Read the model definition and answer for the solid it produces. Units are mm, in the model's axes. Face numbers are marked on the shaded views. A direction names the side the tool comes from. Coordinates: 2 decimals unless noted, no trailing zeros. Write each loop counter-clockwise with the first axis right and the second up, starting at its lowest first coordinate (ties: lowest second). Pieces come first, ordered by that corner, then holes. Notation, with made-up numbers: (-25, 71.5) - (21, 71.5) arc R32 cw to (21, 97.5) - close; hole circle Ø8 at (-12.75, 53). An arc over 180 degrees is marked (long way). Use a Markdown table: item, result.
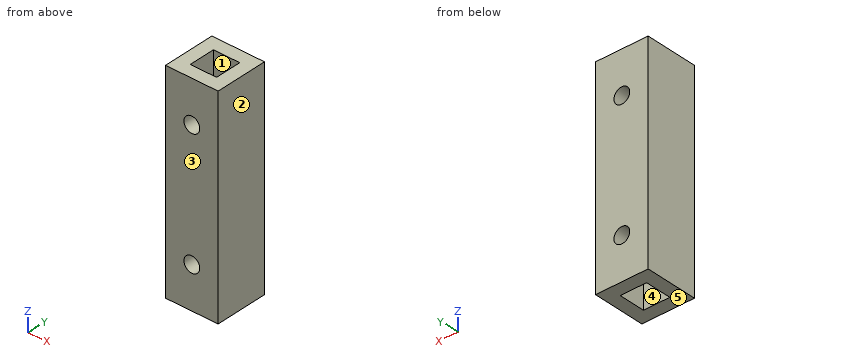
from build123d import *

# Parameters (mm, degrees)
SKETCH_1_W               = 10
SKETCH_1_H               = 10
EXTRUDE_1_DEPTH          = 40
CUT_EXTRUDE_1_DEPTH      = 42.533119315
CUT_EXTRUDE_1_DEPTH_BACK = 42.533119315
SKETCH_2_R               = 1.5
CUT_EXTRUDE_2_DEPTH      = 42.533119315
CUT_EXTRUDE_2_DEPTH_BACK = 42.533119315
SKETCH_3_R               = 1.5
CUT_EXTRUDE_3_DEPTH      = 41.620192023
CUT_EXTRUDE_3_DEPTH_BACK = 41.620192023
SKETCH_4_W               = 5
SKETCH_4_H               = 5


with BuildPart() as part:
    # 草图1 → 凸台-拉伸1 (new body)
    with BuildSketch(Plane.XY):
        Rectangle(SKETCH_1_W, SKETCH_1_H)
    extrude(amount=EXTRUDE_1_DEPTH)

    # 草图2 → 切除-拉伸1 (cut, two sides: drawn at the far end of the back side and taken through both)
    with BuildSketch(Plane(origin=(0, 5, 0), x_dir=(1, 0, 0), z_dir=(0, 1, 0)).offset(-CUT_EXTRUDE_1_DEPTH_BACK)):
        with Locations(Location((0, -8, 0), (0, 0, 270))):
            Circle(SKETCH_2_R)
    extrude(amount=CUT_EXTRUDE_1_DEPTH + CUT_EXTRUDE_1_DEPTH_BACK, mode=Mode.SUBTRACT)

    # 草图3 → 切除-拉伸2 (cut, two sides: drawn at the far end of the back side and taken through both)
    with BuildSketch(Plane(origin=(0, 5, 0), x_dir=(1, 0, 0), z_dir=(0, 1, 0)).offset(-CUT_EXTRUDE_2_DEPTH_BACK)):
        with Locations(Location((0, -32, 0), (0, 0, 270))):
            Circle(SKETCH_3_R)
    extrude(amount=CUT_EXTRUDE_2_DEPTH + CUT_EXTRUDE_2_DEPTH_BACK, mode=Mode.SUBTRACT)

    # 草图4 → 切除-拉伸3 (cut, two sides: drawn at the far end of the back side and taken through both)
    with BuildSketch(Plane.XY.offset(40).offset(-CUT_EXTRUDE_3_DEPTH_BACK)):
        Rectangle(SKETCH_4_W, SKETCH_4_H)
    extrude(amount=CUT_EXTRUDE_3_DEPTH + CUT_EXTRUDE_3_DEPTH_BACK, mode=Mode.SUBTRACT)


solid = part.part
(1) A cutting plane is placed at D-D, the plane y = 3.75. Write down the section's boundary in (x, z), and give its area (3 significant figures).
Report:
| item | result |
|---|---|
| outline | (-5, 0) - (5, 0) - (5, 40) - (-5, 40) - close; hole circle Ø3 at (0, 8); hole circle Ø3 at (0, 32) |
| area | 386 mm² |
(2) A cutting plane is placed at B-B, the plane z = 23. Write down the section's boundary in (x, y), and give its area (3 significant figures).
Report:
| item | result |
|---|---|
| outline | (-5, -5) - (5, -5) - (5, 5) - (-5, 5) - close; hole (-2.5, -2.5) - (2.5, -2.5) - (2.5, 2.5) - (-2.5, 2.5) - close |
| area | 75.0 mm² |
(3) A cutting plane is placed at A-A, the plane y = 1.75. Write down the section's boundary in (x, z), and give its area (3 significant figures).
Report:
| item | result |
|---|---|
| outline | (-5, 0) - (-2.5, 0) - (-2.5, 40) - (-5, 40) - close; (2.5, 0) - (5, 0) - (5, 40) - (2.5, 40) - close |
| area | 200 mm² |
(4) For the marked faces 4 and 5, determine the directions among +Z, -Z, +X, -X, +Y, -Y from which every point of the face is accessible in a straight line to the end or side of a thin tool.
Report:
| item | result |
|---|---|
| face 4 | +Z, -Z |
| face 5 | -Z, +X, -X, +Y, -Y |
(5) A cutting plane is placed at C-C, the plane x = 0. Write down the section's boundary in (y, z), and give its area (3 significant figures).
Report:
| item | result |
|---|---|
| outline | (-5, 0) - (-2.5, 0) - (-2.5, 6.5) - (-5, 6.5) - close; (-5, 9.5) - (-2.5, 9.5) - (-2.5, 30.5) - (-5, 30.5) - close; (-5, 33.5) - (-2.5, 33.5) - (-2.5, 40) - (-5, 40) - close; (2.5, 0) - (5, 0) - (5, 6.5) - (2.5, 6.5) - close; (2.5, 9.5) - (5, 9.5) - (5, 30.5) - (2.5, 30.5) - close; (2.5, 33.5) - (5, 33.5) - (5, 40) - (2.5, 40) - close |
| area | 170 mm² |
(6) Straight lines are drawn through the part: L1, parallel to Z at x = 0, y = 4.3; L2, parallel to Y at x = -1.75, z = 18.5. For each, find the intervals that lie inside material, in ascending order.
Report:
| item | result |
|---|---|
| L1 | z = 0 to 6.5, 9.5 to 30.5, 33.5 to 40 |
| L2 | y = -5 to -2.5, 2.5 to 5 |
(7) The mould has two halves that part along Y. Classify the marked faces 1, 2 and 3: pulls with the +Y half, pulls with the -Y half, needs draft (parallel to the pull), parting line crosses it, or undercut.
Report:
| item | result |
|---|---|
| face 1 | undercut |
| face 2 | needs draft |
| face 3 | pulls with the -Y half |
